Read the model definition and answer for the solid it produces. Units are mm, in the model's axes. A direction names the side the tool comes from. Give positions to 0.01 mm unless a question says otherwise; leave off trailing zeros. Order: outer loops, then holes, each group sorted by start corner. A loop starts at its lowest first (then second) coordinate and runs counter-clockwise, first axis right, second up.
Item 1: Which of the six approach directions +Z, -Z, +X, -X, +Y, -Y give full straight-line access (tool end or side, diameter ignored) to faces 1 (the face through (-2, 2, 2)), 2 (the face through (1.352, 0.993, 4.292))?
Item 2: Find the intervals of material crossed by line 1 along Y through (x, z) = (3, 1.75); line 2 along Z through (x, y) = (0.5, 5); line 3 along Z through (x, y) = (-1, 4.75), in increasing order.
Item 3: A cutting plane is placed at C-C (y = 6.5). Write down the section's boundary in (x, z).
Item 4: A cutting plane is placed at B-B (z = 0). Write down the section's boundary in (x, y).
Item 5: A cutting plane is placed at A-A (x = 0). Write down the section's boundary in (y, z).
from build123d import *

# Parameters (mm, degrees)
SKETCH1_R           = 4.5
SKETCH1_R_2         = 1.6
BOSS_EXTRUDE1_DEPTH = 2
SKETCH1_2_R         = 1.6
BOSS_EXTRUDE2_DEPTH = 8.05
CHAMFER1_SIZE       = 0.7
CHAMFER2_SIZE       = 0.5
CHAMFER3_SIZE       = 0.5


with BuildPart() as part:
    # Sketch1 → Boss-Extrude1 (new body)
    with BuildSketch(Plane(origin=(0, 0, 0), x_dir=(1, 0, 0), z_dir=(0, 1, 0))):
        with Locations(Location((0, 0, 0), (0, 0, 270))):
            Circle(SKETCH1_R)
        with Locations(Location((0, 0, 0), (0, 0, 270))):
            Circle(SKETCH1_R_2, mode=Mode.SUBTRACT)
    extrude(amount=BOSS_EXTRUDE1_DEPTH)

    # Sketch1_2 → Boss-Extrude2 (add)
    with BuildSketch(Plane(origin=(0, 0, 0), x_dir=(1, 0, 0), z_dir=(0, 1, 0))):
        with Locations(Location((0, 0, 0), (0, 0, 270))):
            Circle(SKETCH1_2_R)
    extrude(amount=BOSS_EXTRUDE2_DEPTH)

    # Chamfer1
    chamfer1_edges = [part.edges().sort_by_distance(p)[0] for p in [
        (0, 2, -1.6),
    ]]
    chamfer(chamfer1_edges, length=CHAMFER1_SIZE)

    # Chamfer2
    chamfer2_edges = [part.edges().sort_by_distance(p)[0] for p in [
        (0, 0, -4.5),
        (0, 2, -4.5),
    ]]
    chamfer(chamfer2_edges, length=CHAMFER2_SIZE)

    # Chamfer3
    chamfer3_edges = [part.edges().sort_by_distance(p)[0] for p in [
        (0, 8.05, -1.6),
    ]]
    chamfer(chamfer3_edges, length=CHAMFER3_SIZE)


solid = part.part
Response values:
1. face 1: +Y
1. face 2: +Y, -Y
2. line 1: y = 0 to 2
2. line 2: z = -1.52 to 1.52
2. line 3: z = -1.25 to 1.25
3. outline: circle Ø3.2 at (0, 0)
4. outline: (-4.5, 0.5) - (-4, 0) - (4, 0) - (4.5, 0.5) - (4.5, 1.5) - (4, 2) - (2.3, 2) - (1.6, 2.7) - (1.6, 7.55) - (1.1, 8.05) - (-1.1, 8.05) - (-1.6, 7.55) - (-1.6, 2.7) - (-2.3, 2) - (-4, 2) - (-4.5, 1.5) - close
5. outline: (0, -4) - (0.5, -4.5) - (1.5, -4.5) - (2, -4) - (2, -2.3) - (2.7, -1.6) - (7.55, -1.6) - (8.05, -1.1) - (8.05, 1.1) - (7.55, 1.6) - (2.7, 1.6) - (2, 2.3) - (2, 4) - (1.5, 4.5) - (0.5, 4.5) - (0, 4) - close
